Can you work these out from the model? Positions are in its coordinate system, mm. A direction names the side the tool comes from. Round coordinates to 2 decimals unless told otherwise and drop trailing zeros. Write each loop counter-clockwise with the first axis right and the second up, starting at its lowest first coordinate (ties: lowest second). Pieces come first, ordered by that corner, then holes. Notation, with made-up numbers: (11, -5) - (65, -5) arc R18 cw to (65, 0) - close; hole circle Ø4 at (-35, 19). An arc over 180 degrees is marked (long way). One line per item, written item: value. Start each with the question number.
(1) Thinking about a two-plate mould opening in X: for faces 1 (the face through (-2.9, 30.54, 13.22)), 2 (the face through (0, -3, 10)), 3 (the face through (15, 7, 8)), which applies, +X half, -X half, draft (parallel to the pull), parting line (faces both ways), or undercut?
(2) I want a section at C-C on z = 8.75. List the corners of the cut face in (x, y) for me, plus the area to 3 significant figures.
(3) On a 3-axis mill with a long thin cutter (end or side, diameter ignored), from which of +Z, -Z, +X, -X, +Y, -Y can I reach the whole of each face in a straight line? I mean faces 4 (the face through (0, -21, 5)), 5 (the face through (0, 27.5, 22)). Say none if no direction works.
(4) I want a section at B-B on x = 1.75. List the corners of the cut face in (y, z) for me.
(5) I want a section at A-A on y = -8.5. List the corners of the cut face in (x, z) for me.
(6) I'm going to push flat-ended pins straight in: pin 1 Ø8 at (x, y) = (3, 20) entering from +Z; pin 2 Ø8.5 at (x, z) = (0, 17) entering from +Y; pin 3 Ø10 at (x, z) = (-2.5, 21) entering from -Y. Where does each tip first touch, or does it pass through?
(7) I want a section at D-D on z = 15.5. List the corners of the cut face in (x, y) for me, plus the area to 3 significant figures.
(8) If I drill on L1, parallel to X at y = 30.45, z = 17 (3 decimals); L2, parallel to Y at x = -0.75, z = 9.5; L3, parallel to Y at x = -8.5, z = 13.75, over which ranges is the centre line in solid material (lowest first)? Write a range as from..to.
from build123d import *

# Parameters (mm, degrees)
ESBO_O1_W                = 30
ESBO_O1_H                = 67
RESSALTO_EXTRUS_O1_DEPTH = 10
ESBO_O2_W                = 30
ESBO_O2_H                = 6
RESSALTO_EXTRUS_O2_DEPTH = 20
CORTE_EXTRUS_O1_REACH    = 76.927
ESBO_O3_R                = 4.765
ESBO_O4_R                = 2.5
CORTE_EXTRUS_O2_DEPTH    = 10


with BuildPart() as part:
    # Esboço1 → Ressalto-extrusão1 (new body)
    with BuildSketch(Plane.XY):
        Rectangle(ESBO_O1_W, ESBO_O1_H)
    extrude(amount=RESSALTO_EXTRUS_O1_DEPTH)

    # Esboço2 → Ressalto-extrusão2 (add)
    with BuildSketch(Plane.XY.offset(10)):
        with Locations((0, 30.5)):
            Rectangle(ESBO_O2_W, ESBO_O2_H)
    extrude(amount=RESSALTO_EXTRUS_O2_DEPTH)

    # Esboço3 → Corte-extrusão1 (cut, up to next)
    with BuildSketch(Plane(origin=(0, 33.5, 0), x_dir=(1, 0, 0), z_dir=(0, 1, 0)), mode=Mode.PRIVATE) as corte_extrus_o1_sk1:
        with Locations(Location((0, -17, 0), (0, 0, 270))):
            Circle(ESBO_O3_R)
    corte_extrus_o1_tool1 = extrude(corte_extrus_o1_sk1.sketch, amount=-CORTE_EXTRUS_O1_REACH, mode=Mode.PRIVATE) & part.part
    add(corte_extrus_o1_tool1.solids().sort_by_distance((0, 33.5, 17))[0], mode=Mode.SUBTRACT)

    # Esboço4 → Corte-extrusão2 (cut)
    with BuildSketch(Plane(origin=(0, 0, 0), x_dir=(-1, 0, 0), z_dir=(0, 0, -1))):
        with Locations((0, -23.5)):
            Circle(ESBO_O4_R)
        with Locations((0, -8.5)):
            Circle(ESBO_O4_R)
    extrude(amount=-CORTE_EXTRUS_O2_DEPTH, mode=Mode.SUBTRACT)


solid = part.part
Established:
1. face 1: undercut
1. face 2: draft
1. face 3: +X half
2. outline: (-15, -33.5) - (15, -33.5) - (15, 33.5) - (-15, 33.5) - close; hole circle Ø5 at (0, -23.5); hole circle Ø5 at (0, -8.5)
2. area: 1,970 mm2
3. face 4: +Z, -Z
3. face 5: +Z, +X, -X, -Y
4. outline: (-33.5, 0) - (-25.29, 0) - (-25.29, 10) - (-33.5, 10) - close; (-21.71, 0) - (-10.29, 0) - (-10.29, 10) - (-21.71, 10) - close; (-6.71, 0) - (33.5, 0) - (33.5, 12.57) - (27.5, 12.57) - (27.5, 10) - (-6.71, 10) - close; (27.5, 21.43) - (33.5, 21.43) - (33.5, 30) - (27.5, 30) - close
5. outline: (-15, 0) - (-2.5, 0) - (-2.5, 10) - (-15, 10) - close; (2.5, 0) - (15, 0) - (15, 10) - (2.5, 10) - close
6. pin 1: z = 10
6. pin 2: through
6. pin 3: y = 27.5
7. outline: (-15, 27.5) - (-4.52, 27.5) - (-4.52, 33.5) - (-15, 33.5) - close; (4.52, 27.5) - (15, 27.5) - (15, 33.5) - (4.52, 33.5) - close
7. area: 126 mm2
8. L1: -15..-4.765, 4.765..15
8. L2: -33.5..-25.88, -21.12..-10.88, -6.12..33.5
8. L3: 27.5..33.5
